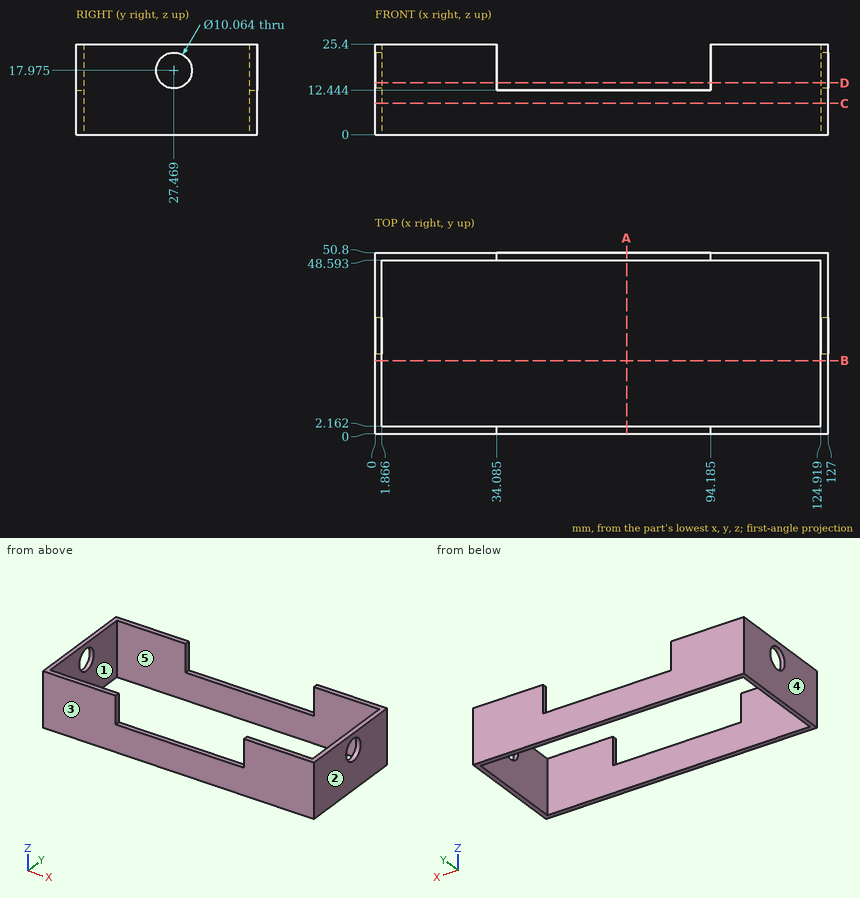
Study the drawing (mm; zero at the part's minimum x, y, z) and answer. A direction names the side the tool comes from. Give positions to 0.01 mm unless a question says otherwise; leave off trailing zeros. Loops run counter-clockwise (first coordinate to the right, second up) from the corner with the lowest first, then second, coordinate; pieces in that order, holes last. Notation, with made-up numbers: M 81.25,-21.5 L 126.25,-21.5 A29 cw 126.25,11.5 Z; hole C 84.25,65.5 d11. An arc over 180 degrees is marked long. One line per item, written item: value. Start each with the question number.
1. This flat-tipped pin is pushed along its axis until it touches: P1, Ø1.7, axis at x = 71.5, y = 1, coming from the +Z side. Where does it stop, or does it pass through?
2. Find section C-C (z = 8.75). Give the vertices of the cut face in (x, y).
3. Which of the six approach directions +Z, -Z, +X, -X, +Y, -Y give full straight-line access (tool end or side, diameter ignored) to the marked faces 1 and 2?
4. Find section D-D (z = 14.5). Give the vertices of the cut face in (x, y) (1 decimal).
5. Find section B-B (y = 20.5). Give the vertices of the cut face in (x, z), and give its area (3 significant figures).
6. Find section A-A (x = 70.5). Give the vertices of the cut face in (y, z).
7. Determine the mould class of the marked faces 3, 4 and 5 for opening direction X: released by +X, released by -X, zero draft, split by the parting line, or undercut.
8. Find the intervals of material crossed by probe 1 along Y at (x, z) = (33.5, 23); probe 2 along X at (y, z) = (22.5, 22.5), in increasing order.
Reported:
1. P1: stops at z = 12.44
2. outline: M 0,0 L 127,0 L 127,50.8 L 0,50.8 Z; hole M 1.87,2.16 L 124.92,2.16 L 124.92,48.59 L 1.87,48.59 Z
3. face 1: +Z, -Z
3. face 2: +Z, -Z, +X, +Y, -Y
4. outline: M 0,0 L 34.1,0 L 34.1,2.2 L 1.9,2.2 L 1.9,23.8 L 0,23.8 Z; M 0,31.1 L 1.9,31.1 L 1.9,48.6 L 34.1,48.6 L 34.1,50.8 L 0,50.8 Z; M 94.2,0 L 127,0 L 127,23.8 L 124.9,23.8 L 124.9,2.2 L 94.2,2.2 Z; M 94.2,48.6 L 124.9,48.6 L 124.9,31.1 L 127,31.1 L 127,50.8 L 94.2,50.8 Z
5. outline: M 0,0 L 1.87,0 L 1.87,25.4 L 0,25.4 Z; M 124.92,0 L 127,0 L 127,25.4 L 124.92,25.4 Z
5. area: 100 mm²
6. outline: M 0,0 L 2.16,0 L 2.16,12.44 L 0,12.44 Z; M 48.59,0 L 50.8,0 L 50.8,12.44 L 48.59,12.44 Z
7. face 3: zero draft
7. face 4: released by -X
7. face 5: undercut
8. probe 1: y = 0 to 2.16, 48.59 to 50.8
8. probe 2: x = 0 to 1.87, 124.92 to 127
